from build123d import *

# Parameters (mm, degrees)
F1_DEPTH = 63.5
F2_DEPTH = 25.4
F3_DEPTH = 7.9375
F0_W     = 25.4
F0_H     = 19.05
F4_DEPTH = 25.4
F6_R     = 6.35


with BuildPart() as f1:
    # F0 (on Front) → F1 (new body, symmetric)
    with BuildSketch(Plane.XZ):
        Polygon((41.275, -9.525), (41.275, 9.525), (22.225, 9.525), (-41.275, 9.525), (-41.275, -9.525), align=None)
    extrude(amount=F1_DEPTH, both=True)

    # F0 (on Front) → F2 (join, symmetric)
    with BuildSketch(Plane.XZ):
        with BuildLine():
            Line((22.225, 9.525), (41.275, 9.525))
            Line((41.275, 9.525), (41.275, 27.0002))
            ThreePointArc((41.275, 27.0002), (45.9246798487, 38.2255201513), (57.15, 42.8752))
            Line((57.15, 42.8752), (84.7223362398, 42.8752))
            Line((84.7223362398, 42.8752), (84.7223362398, 61.9252))
            Line((84.7223362398, 61.9252), (57.15, 61.9252))
            ThreePointArc((57.15, 61.9252), (32.4542956671, 51.6959043329), (22.225, 27.0002))
            Line((22.225, 27.0002), (22.225, 9.525))
        make_face()
    extrude(amount=F2_DEPTH, both=True)

    # F0 (on Front) → F3 (join, symmetric)
    with BuildSketch(Plane.XZ):
        with BuildLine():
            Line((-41.275, 9.525), (22.225, 9.525))
            Line((22.225, 9.525), (22.225, 27.0002))
            ThreePointArc((22.225, 27.0002), (32.4542956671, 51.6959043329), (57.15, 61.9252))
            add(Edge.make_bspline(
                [(-41.275, 9.525), (-31.9519031348, 41.2950287538), (16.3025462672, 64.0494193526), (57.15, 61.9252)],
                knots=[0, 0, 0, 0, 111.5045361635, 111.5045361635, 111.5045361635, 111.5045361635], degree=3))
        make_face()
    extrude(amount=F3_DEPTH, both=True)

    # F0 (on Front) → F4 (join, symmetric)
    with BuildSketch(Plane.XZ):
        with Locations((97.4223362398, 52.4002)):
            Rectangle(F0_W, F0_H)
    extrude(amount=F4_DEPTH, both=True)

    # F0 (on Front) → F5 (revolve)
    with BuildSketch(Plane.XZ):
        Polygon((110.1223362398, 61.9252), (110.1223362398, 42.8752), (110.1223362398, 38.1), (135.5223362398, 38.1), (135.5223362398, 66.675), (110.1223362398, 66.675), align=None)
    revolve(axis=Axis((110.1223362398, 0, 52.3875), (0, 0, 1)))

    # F6
    f6_edges = [f1.edges().sort_by_distance(p)[0] for p in [
        (-41.275, -63.5, 0),
        (41.275, -63.5, 0),
        (41.275, 63.5, 0),
        (-41.275, 63.5, 0),
    ]]
    fillet(f6_edges, radius=F6_R)


solid = f1.part
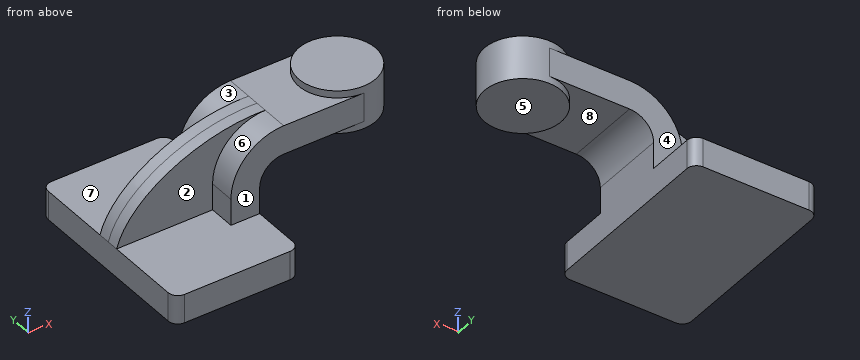
For this review, take the finished solid that the model builds, in its own axes (mm). Face numbers are marked on the shaded views. A direction names the side the tool comes from. Round coordinates to 2 decimals unless told otherwise and drop trailing zeros. Loops run counter-clockwise (first coordinate to the right, second up) from the corner with the lowest first, then second, coordinate; pieces in that order, holes last. Notation, with made-up numbers: (30.5, 88) - (77.5, 88) arc R26 cw to (77.5, 121) - close; hole circle Ø3 at (13, 49). An arc over 180 degrees is marked (long way). Use one line per item in the form item = value.
Item 1: Clearance check with flat-ended pins moving along their axes: P1, Ø1, axis at x = -16.5, y = 9.5, coming from the +Z side (3 decimals); P2, Ø15.5, axis at x = 73, z = 36, coming from the +Y side; P3, Ø12, axis at x = 46, y = -5.5, coming from the +Z side. State where each tip first meets the part, or that it passes through.
Answers:
P1 = 9.525
P2 = 25.4
P3 = 62.06
Item 2: Consider section B-B on y = 47.5. Write out the cut boundary in (x, z) (3 decimals).
Answers:
outline = (-41.275, -9.525) - (41.275, -9.525) - (41.275, 9.525) - (-41.275, 9.525) - close
Item 3: Mouldability with a two-part tool opening along X and no side actions: class the marked faces 6, 7 and 8 as +X half, -X half, draft (parallel to the pull), parting line (faces both ways), or undercut.
Answers:
face_6 = -X half
face_7 = draft
face_8 = undercut
Item 4: Tool access review of the marked faces 1, 2, 3, 4 and 5: name each direction out of +Z, -Z, +X, -X, +Y, -Y from which nothing blocks a thin tool from reaching the whole face with its end or side.
Answers:
face_1 = +Z, +X, -X, -Y
face_2 = +Z, -X, -Y
face_3 = +Z, -X, +Y
face_4 = +Z, +X, -X, +Y
face_5 = -Z, +X, +Y, -Y
Item 5: For line 1 (Z direction, x = 127, y = -3) (3 decimals); line 2 (Y direction, x = 19.5, z = 18.5); line 3 (X direction, y = -16.5, z = 26) (3 decimals), list the stretches that pass through material, from the lowest coordinate up.
Answers:
line_1 = 38.1 to 66.675
line_2 = -7.94 to 7.94
line_3 = 22.225 to 41.275
Item 6: Consider section A-A on y = 21.5. Write out the cut boundary in (x, z) (3 decimals), then the cut area to 3 significant figures.
Answers:
outline = (-41.275, -9.525) - (41.275, -9.525) - (41.275, 27) arc R15.875 cw to (57.15, 42.875) - (96.598, 42.875) - (96.598, 38.1) - (123.647, 38.1) - (123.647, 66.675) - (96.598, 66.675) - (96.598, 61.925) - (57.15, 61.925) arc R34.925 ccw to (22.225, 27) - (22.225, 9.525) - (-41.275, 9.525) - close
area = 4,190 mm^2
